from build123d import *

# Parameters (mm, degrees)
CUT_EXTRUDE1_DEPTH = 38.422447809
CUT_EXTRUDE2_START = 5.5
CUT_EXTRUDE2_DEPTH = 32.922447809
SKETCH4_R          = 1.1
SKETCH4_R_2        = 4.245
CUT_EXTRUDE3_DEPTH = 38.422447874


with BuildPart() as part:
    # Sketch1 → Revolve1 (revolve)
    with BuildSketch(Plane(origin=(0, 0, 0), x_dir=(1, 0, 0), z_dir=(0, 1, 0)), mode=Mode.PRIVATE) as revolve1_sk:
        Polygon((-14, 0), (-14, 14.14), (-18, 14.14), (-18, 12.57), (-24.5, 12.57), (-24.5, 11), (-18, 11), (-18, 9.43), (-24.5, 9.43), (-24.5, 4.71), (-18, 4.71), (-18, 3.14), (-24.5, 3.14), (-24.5, 1.57), (-18, 1.57), (-18, 0), align=None)
    revolve(revolve1_sk.sketch.rotate(Axis((0, 0, 0), (0, 0, -1)), 180), axis=Axis((0, 0, 0), (0, 0, -1)))

    # Sketch2 → Cut-Extrude1 (cut, through all)
    with BuildSketch(Plane.XY):
        with BuildLine():
            Line((-24.5, 0), (24.5, 0))
            ThreePointArc((24.5, 0), (0, -24.5), (-24.5, 0))
        make_face()
    extrude(amount=-CUT_EXTRUDE1_DEPTH, mode=Mode.SUBTRACT)

    # Sketch3 → Cut-Extrude2 (cut, through all)
    with BuildSketch(Plane(origin=(0, 0, 0), x_dir=(1, 0, 0), z_dir=(0, 1, 0)).offset(CUT_EXTRUDE2_START)):
        with BuildLine():
            Line((-23.584646978, 9.43), (-24.5, 9.43))
            Line((-24.5, 9.43), (-24.5, 4.71))
            Line((-24.5, 4.71), (-23.584646978, 4.71))
            ThreePointArc((-23.584646978, 4.71), (-17.5, 7.07), (-23.584646978, 9.43))
        make_face()
        with BuildLine():
            Line((23.584646978, 4.71), (24.5, 4.71))
            Line((24.5, 4.71), (24.5, 9.43))
            Line((24.5, 9.43), (23.584646978, 9.43))
            ThreePointArc((23.584646978, 9.43), (17.5, 7.07), (23.584646978, 4.71))
        make_face()
    extrude(amount=CUT_EXTRUDE2_DEPTH, mode=Mode.SUBTRACT)

    # Sketch4 → Cut-Extrude3 (cut, through all)
    with BuildSketch(Plane.XZ):
        with Locations(Location((-21, -7.07, 0), (0, 0, 270))):
            Circle(SKETCH4_R)
        with Locations(Location((21, -7.07, 0), (0, 0, 270))):
            Circle(SKETCH4_R)
        with Locations(Location((0, -7.07, 0), (0, 0, 270))):
            Circle(SKETCH4_R_2)
    extrude(amount=-CUT_EXTRUDE3_DEPTH, mode=Mode.SUBTRACT)


solid = part.part
Read the model definition and answer for the solid it produces. Units are mm, in the model's axes. A direction names the side the tool comes from. Round coordinates to 2 decimals unless told otherwise and drop trailing zeros. Write each loop counter-clockwise with the first axis right and the second up, starting at its lowest first coordinate (ties: lowest second). Pieces come first, ordered by that corner, then holes. Notation, with made-up numbers: M -38.5,-33 L 18.5,-33 A29 cw 18.5,-12 Z; hole C 5,-28.5 d9. An arc over 180 degrees is marked long. Use a Markdown table: item, result.
1) The part is cut by section D-D (y = 4.75). Give the number of separate pieces and of enclosed holes in the cut face, plus the area to 3 significant figures.
Answers follow:
| item | result |
|---|---|
| separate pieces | 2 |
| enclosed holes | 2 |
| area | 216 mm2 |
2) For a pull along X with two mould halves and no side action, classify faces 1 (the cylindrical face through (-22.074, 2.712, -6.832)), 2 (the flat face through (-16, 12, -11)), 3 (the cylindrical face through (-0.539, 24.494, -2.344)) as pulls with the +X half, pulls with the -X half, needs draft (parallel to the pull), parting line crosses it, or undercut.
Answers follow:
| item | result |
|---|---|
| face 1 | undercut |
| face 2 | needs draft |
| face 3 | parting line crosses it |
3) The part is cut by section C-C (z = -7.25). Write down the section's boundary in (x, y).
Answers follow:
| item | result |
|---|---|
| outline | M -24.5,0 L -22.09,0 L -22.09,5.5 L -23.87,5.5 A24.5 ccw Z; M -19.91,0 L -14,0 A14 cw -4.24,13.34 L -4.24,24.13 A24.5 ccw -17.5,17.14 L -17.5,5.5 L -19.91,5.5 Z; M 4.24,13.34 A14 cw 14,0 L 19.91,0 L 19.91,5.5 L 17.5,5.5 L 17.5,17.14 A24.5 ccw 4.24,24.13 Z; M 22.09,0 L 24.5,0 A24.5 ccw 23.87,5.5 L 22.09,5.5 Z |
4) The part is cut by section A-A (y = 19). Write down the section's boundary in (x, z) (3 decimals), plus the area to 3 significant figures.
Answers follow:
| item | result |
|---|---|
| outline | M -15.468,-12.57 L 15.468,-12.57 L 15.468,-11 L 1.605,-11 A4.245 cw -1.605,-11 L -15.468,-11 Z; M -15.468,-9.43 L -3.529,-9.43 A4.245 cw -3.529,-4.71 L -15.468,-4.71 Z; M -15.468,-3.14 L -1.605,-3.14 A4.245 cw 1.605,-3.14 L 15.468,-3.14 L 15.468,-1.57 L -15.468,-1.57 Z; M 3.529,-9.43 L 15.468,-9.43 L 15.468,-4.71 L 3.529,-4.71 A4.245 cw Z |
| area | 204 mm2 |
5) A tool of negligible diameter and unlimited length cuts with its end or side. For faces 4 (the flat face through (14, 13, -4.71)), 5 (the flat face through (0, 20, -1.57)), 6 (the cylindrical face through (0, 18, -13)), 7 (the flat face through (-14, 13, -4.71)), from which of +Z, -Z, +X, -X, +Y, -Y can it reach the whole face along a straight path? Write none if from no direction.
Answers follow:
| item | result |
|---|---|
| face 4 | +X, +Y |
| face 5 | +Z, +Y |
| face 6 | -Z, +Y |
| face 7 | -X, +Y |
6) Flat-ended cylindrical pins translate along their axes: pin 1 (8 mm diameter, centred on x = -8, z = -6.5, fed in from +Y); pin 2 (3.5 mm diameter, centred on x = 21, z = -7.07, fed in from +Y); pin 3 (6 mm diameter, centred on y = 6.5, z = -1.5, fed in from +X). Find the tip coordinate at first contact, or state that the pin passes through.
Answers follow:
| item | result |
|---|---|
| pin 1 | stops at y = 24.16 |
| pin 2 | stops at y = 5.5 |
| pin 3 | stops at x = 24.25 |
7) The part is cut by section B-B (x = 0). Write down the section's boundary in (y, z) (3 decimals), plus the area to 3 significant figures.
Answers follow:
| item | result |
|---|---|
| outline | M 14,-14.14 L 18,-14.14 L 18,-12.57 L 24.5,-12.57 L 24.5,-11.315 L 14,-11.315 Z; M 14,-2.825 L 24.5,-2.825 L 24.5,-1.57 L 18,-1.57 L 18,0 L 14,0 Z |
| area | 38.9 mm2 |
8) Straight lines are drawn through the part: line 1 along X through (y, z) = (1.8, -7.07); line 2 along X through (y, z) = (3.1, -7.07); line 3 along Z through (x, y) = (0, 16.25) (3 decimals). For each, find the intervals that lie inside material, in ascending order. Write a range as [from, to].
Answers follow:
| item | result |
|---|---|
| line 1 | x = [-24.43, -22.1], [-19.9, -13.88], [13.88, 19.9], [22.1, 24.43] |
| line 2 | x = [-24.3, -22.1], [-19.9, -13.65], [13.65, 19.9], [22.1, 24.3] |
| line 3 | z = [-14.14, -11.315], [-2.825, 0] |
